from build123d import *

# Parameters (mm, degrees)
BOSS_EXTRUDE1_DEPTH     = 7.2
SKETCH2_R               = 1.61
BOSS_EXTRUDE2_DEPTH     = 1.5
BOSS_EXTRUDE3_DEPTH     = 0.7
BOSS_EXTRUDE7_DEPTH     = 4.22
CUT_EXTRUDE1_DEPTH      = 7.544999991
CUT_EXTRUDE1_DEPTH_BACK = 7.544999991
ESQUISSE1_W             = 29.65
ESQUISSE1_H             = 9.089999982
BOSS_EXTRU_1_DEPTH      = 4.5
ESQUISSE3_W             = 16
ESQUISSE3_H             = 7.089999982
ESQUISSE3_W_2           = 7
BOSS_EXTRU_2_DEPTH      = 2
ESQUISSE4_R             = 3
ESQUISSE4_W             = 15.2
ESQUISSE4_H             = 6.289999982
ENL_V_MAT_EXTRU_1_DEPTH = 2
ESQUISSE5_W             = 8.71
ESQUISSE5_H             = 1
BOSS_EXTRU_3_DEPTH      = 8
BOSS_EXTRU_4_DEPTH      = 8


with BuildPart() as part:
    # Sketch1 → Boss-Extrude1 (new body)
    with BuildSketch(Plane(origin=(0, 0, 0), x_dir=(1, 0, 0), z_dir=(0, 1, 0))):
        Polygon((-14.055, 5.774999991), (-5.355, 5.774999991), (-5.355, 6.544999991), (-14.825, 6.544999991), (-14.825, -6.544999991), (14.825, -6.544999991), (14.825, 6.544999991), (5.355, 6.544999991), (5.355, 5.774999991), (14.055, 5.774999991), (14.055, -5.774999991), (-14.055, -5.774999991), align=None)
    extrude(amount=BOSS_EXTRUDE1_DEPTH)

    # Sketch2 → Boss-Extrude2 (add)
    with BuildSketch(Plane(origin=(0, 0, 0), x_dir=(1, 0, 0), z_dir=(0, 1, 0))):
        with BuildLine():
            Line((18.64, 3.735), (14.825, 3.735))
            Line((14.825, 3.735), (14.825, -3.735))
            Line((14.825, -3.735), (18.64, -3.735))
            ThreePointArc((18.64, -3.735), (22.375, 0), (18.64, 3.735))
        make_face()
        with Locations((18.64, 0)):
            Circle(SKETCH2_R, mode=Mode.SUBTRACT)
        with BuildLine():
            Line((-14.825, 3.735), (-14.825, -3.735))
            Line((-14.825, -3.735), (-18.64, -3.735))
            ThreePointArc((-18.64, -3.735), (-22.375, 0), (-18.64, 3.735))
            Line((-18.64, 3.735), (-14.825, 3.735))
        make_face()
        with Locations((-18.64, 0)):
            Circle(SKETCH2_R, mode=Mode.SUBTRACT)
    extrude(amount=BOSS_EXTRUDE2_DEPTH)

    # Sketch3 → Boss-Extrude3 (add)
    with BuildSketch(Plane(origin=(0, 7.2, 0), x_dir=(1, 0, 0), z_dir=(0, 1, 0))):
        Polygon((-14.825, -6.544999991), (14.825, -6.544999991), (14.825, 6.544999991), (5.355, 6.544999991), (5.355, 4.324999991), (-5.355, 4.324999991), (-5.355, 6.544999991), (-14.825, 6.544999991), align=None)
    extrude(amount=-BOSS_EXTRUDE3_DEPTH)

    # Sketch7 → Boss-Extrude7 (add)
    with BuildSketch(Plane(origin=(0, 1.5, 0), x_dir=(1, 0, 0), z_dir=(0, 1, 0))):
        with BuildLine():
            Line((-14.825, 3.735), (-16.625, 3.735))
            ThreePointArc((-16.625, 3.735), (-15.518302355, 2.690023234), (-14.825, 1.335))
            Line((-14.825, 1.335), (-14.825, 3.735))
        make_face()
        with BuildLine():
            Line((-14.825, -3.735), (-14.825, -1.335))
            ThreePointArc((-14.825, -1.335), (-15.518302355, -2.690023234), (-16.625, -3.735))
            Line((-16.625, -3.735), (-14.825, -3.735))
        make_face()
        with BuildLine():
            Line((14.825, -3.735), (16.625, -3.735))
            ThreePointArc((16.625, -3.735), (15.518302355, -2.690023234), (14.825, -1.335))
            Line((14.825, -1.335), (14.825, -3.735))
        make_face()
        with BuildLine():
            Line((14.825, 3.735), (14.825, 1.335))
            ThreePointArc((14.825, 1.335), (15.518302355, 2.690023234), (16.625, 3.735))
            Line((16.625, 3.735), (14.825, 3.735))
        make_face()
    extrude(amount=BOSS_EXTRUDE7_DEPTH)

    # Sketch8 → Cut-Extrude1 (cut, two sides)
    with BuildSketch(Plane.XY) as cut_extrude1_sk:
        Polygon((-14.825, 5.72), (-16.625, 3.92), (-16.625, 5.72), align=None)
        Polygon((14.825, 5.72), (16.625, 3.92), (16.625, 5.72), align=None)
    extrude(amount=CUT_EXTRUDE1_DEPTH, mode=Mode.SUBTRACT)
    extrude(cut_extrude1_sk.sketch, amount=-CUT_EXTRUDE1_DEPTH_BACK, mode=Mode.SUBTRACT)

    # Esquisse1 → Boss.-Extru.1 (add)
    with BuildSketch(Plane(origin=(0, 7.2, 0), x_dir=(1, 0, 0), z_dir=(0, 1, 0))):
        Rectangle(ESQUISSE1_W, ESQUISSE1_H)
    extrude(amount=BOSS_EXTRU_1_DEPTH)

    # Esquisse3 → Boss.-Extru.2 (add)
    with BuildSketch(Plane(origin=(0, 11.7, 0), x_dir=(1, 0, 0), z_dir=(0, 1, 0))):
        with Locations((-5.825, 0)):
            Rectangle(ESQUISSE3_W, ESQUISSE3_H)
        with Locations((10.325, 0)):
            Rectangle(ESQUISSE3_W_2, ESQUISSE3_H)
    extrude(amount=BOSS_EXTRU_2_DEPTH)

    # Esquisse4 → Enlèv. mat.-Extru.1 (cut)
    with BuildSketch(Plane(origin=(0, 13.7, 0), x_dir=(1, 0, 0), z_dir=(0, 1, 0))):
        with Locations((10.325, 0)):
            Circle(ESQUISSE4_R)
        with Locations((-5.825, 0)):
            Rectangle(ESQUISSE4_W, ESQUISSE4_H)
    extrude(amount=-ENL_V_MAT_EXTRU_1_DEPTH, mode=Mode.SUBTRACT)

    # Esquisse5 → Boss.-Extru.3 (add)
    with BuildSketch(Plane.XZ.offset(-6.5)):
        with Locations((0, -4.044999991)):
            Rectangle(ESQUISSE5_W, ESQUISSE5_H)
    extrude(amount=BOSS_EXTRU_3_DEPTH)

    # Esquisse6 → Boss.-Extru.4 (add)
    with BuildSketch(Plane(origin=(0, 0, -4.544999991), x_dir=(-1, 0, 0), z_dir=(0, 0, -1))):
        Polygon((-4.355, -1.5), (-3.355, -1.5), (-3.355, 5.5), (3.355, 5.5), (3.355, -1.5), (4.355, -1.5), (4.355, 6.5), (-4.355, 6.5), align=None)
    extrude(amount=BOSS_EXTRU_4_DEPTH)


solid = part.part
Design review of the part built by this model. Coordinates are the model's own, in mm. A direction names the side the tool comes from. Round coordinates to 2 decimals unless told otherwise and drop trailing zeros. Write each loop counter-clockwise with the first axis right and the second up, starting at its lowest first coordinate (ties: lowest second). Pieces come first, ordered by that corner, then holes. Notation, with made-up numbers: M 16.25,-5 L 44.25,-5 A24 ccw 44.25,11 Z; hole C 69.5,54.5 d7. An arc over 180 degrees is marked long. One line per item, written item: value. Start each with the question number.
1. To check wall thickness, follow probe 1 along X at (y, z) = (1.1, 0) (3 decimals); probe 2 along Z at (x, y) = (-18.64, 0.5) (3 decimals); probe 3 along Z at (x, y) = (-6.5, 12.5) (3 decimals). State the ranges of each line that lie inside material, in increasing order. Write a range as from..to.
2. For faces 1 (the face through (2.175, 13, 0)), 2 (the face through (0, 2, -4.545)), 3 (the face through (-16.87, 1.5, -0.05)), 4 (the face through (-6, 13, 3.545)), list the 3-axis set-ups (+Z, -Z, +X, -X, +Y, -Y) from which the entire face can be reached by the end or side of a thin tool; tool diameter is ignored.
3. Clearance check with flat-ended pins moving along their axes: P1, Ø10.5, axis at x = -10, z = 1.5, coming from the -Y side; P2, Ø1, axis at x = -8.5, y = 12.5, coming from the +Z side (3 decimals); P3, Ø0.6, axis at x = -8.5, z = -5.5, coming from the +Y side. State where each tip first meets the part, or that it passes through.
4. Take a section at C-C on z = 0. State how many separate pieces and enclosed holes the cut face has, then the cut area to 3 significant figures.
5. Take a section at B-B on x = 6. State the section outline as (y, z) points (3 decimals), then the cut area to 3 significant figures.
6. Draft analysis for pull direction X (two halves, no side actions). For faces 5 (the face through (-15.312, 5.233, 3.052)), 6 (the face through (10, 3, -5.775)), 7 (the face through (0, 4, 6.545)), 8 (the face through (5.355, 4, -6)), state which applies: pulls with the +X half, pulls with the -X half, needs draft (parallel to the pull), parting line crosses it, or undercut.
Computed:
1. probe 1: x = -22.375..-20.25, -17.03..-14.055, 14.055..17.03, 20.25..22.375
1. probe 2: z = -3.735..-1.61, 1.61..3.735
1. probe 3: z = -3.545..-3.145, 3.145..3.545
2. face 1: +Z, -Z, +Y
2. face 2: -Z, -Y
2. face 3: -X, +Y
2. face 4: +Z, +X, -X, +Y
3. P1: stops at y = 0
3. P2: stops at z = 3.545
3. P3: stops at y = 7.2
4. separate pieces: 3
4. enclosed holes: 0
4. area: 181 mm²
5. outline: M 0,-6.545 L 7.2,-6.545 L 7.2,-4.545 L 11.7,-4.545 L 11.7,4.545 L 7.2,4.545 L 7.2,6.545 L 0,6.545 L 0,5.775 L 6.5,5.775 L 6.5,-5.775 L 0,-5.775 Z
5. area: 60.1 mm²
6. face 5: pulls with the -X half
6. face 6: undercut
6. face 7: needs draft
6. face 8: undercut
